Read the model definition and answer for the solid it produces. Units are mm, in the model's axes. A direction names the side the tool comes from. Give positions to 0.01 mm unless a question says otherwise; leave off trailing zeros. Order: outer loops, then holes, each group sorted by start corner. A loop starts at its lowest first (then second) coordinate and runs counter-clockwise, first axis right, second up.
Item 1: The mould has two halves that part along Z. Classify faces 1 (the face through (11.623, 3.738, -2.581)), 2 (the face through (8, 5.556, -4)), 3 (the face through (-3.86, 4.83, -5.04)): +Z half, -Z half, draft (parallel to the pull), parting line (faces both ways), or undercut.
Item 2: Given pin 1 Ø1 at (x, y) = (0, 8) entering from +Z; pin 2 Ø1 at (x, y) = (-7, 7) entering from +Z, each flat-ended and moving along its own axis, determine where each tip first touches the part or whether it passes through.
Item 3: A cutting plane is placed at D-D (y = 7.5). Write down the section's boundary in (x, z), plus the area to 3 significant figures.
Item 4: A cutting plane is placed at A-A (x = 0). Write down the section's boundary in (y, z) (3 decimals), plus the area to 3 significant figures.
Item 5: A cutting plane is placed at B-B (z = 0). Write down the section's boundary in (x, y) (3 decimals).
Item 6: A cutting plane is placed at C-C (y = 5). Write down the section's boundary in (x, z), plus the area to 3 significant figures.
Item 7: Which of the six approach directions +Z, -Z, +X, -X, +Y, -Y give full straight-line access (tool end or side, diameter ignored) to faces 4 (the face through (8.524, 4.751, 1.893)), 5 (the face through (-6, 0, 3))?
Item 8: Find the intervals of material crossed by line 1 along X through (y, z) = (4, 0); line 2 along X through (y, z) = (3.5, 0); line 3 along Y through (x, z) = (-4, 9.5), in increasing order.
from build123d import *

# Parameters (mm, degrees)
SKETCH1_R           = 8.73125
BOSS_EXTRUDE1_DEPTH = 9.525
SKETCH3_R           = 11.90625
BOSS_EXTRUDE2_DEPTH = 3.96875
BOSS_EXTRUDE3_START = -3.96875
SKETCH4_R           = 11.90625
BOSS_EXTRUDE3_DEPTH = 3.96875
SKETCH2_R           = 6.35
CUT_EXTRUDE2_DEPTH  = 20.345366451
FILLET2_R           = 3.5


with BuildPart() as part:
    # Sketch1 → Boss-Extrude1 (new body)
    with BuildSketch(Plane(origin=(0, 0, 0), x_dir=(1, 0, 0), z_dir=(0, 1, 0))):
        with Locations(Location((0, 0, 0), (0, 0, 90))):
            Circle(SKETCH1_R)
    extrude(amount=BOSS_EXTRUDE1_DEPTH)

    # Sketch3 → Boss-Extrude2 (add)
    with BuildSketch(Plane(origin=(0, 9.525, 0), x_dir=(1, 0, 0), z_dir=(0, 1, 0))):
        with Locations(Location((0, 0, 0), (0, 0, 270))):
            Circle(SKETCH3_R)
    extrude(amount=-BOSS_EXTRUDE2_DEPTH)

    # Sketch4 → Boss-Extrude3 (add)
    with BuildSketch(Plane(origin=(0, 0, 0), x_dir=(-1, 0, 0), z_dir=(0, -1, 0)).offset(BOSS_EXTRUDE3_START)):
        with Locations(Location((0, 0, 0), (0, 0, 270))):
            Circle(SKETCH4_R)
    extrude(amount=BOSS_EXTRUDE3_DEPTH)

    # Sketch2 → Cut-Extrude2 (cut, through all)
    with BuildSketch(Plane(origin=(0, 9.525, 0), x_dir=(1, 0, 0), z_dir=(0, 1, 0))):
        with Locations(Location((0, 0, 0), (0, 0, 270))):
            Circle(SKETCH2_R)
    extrude(amount=-CUT_EXTRUDE2_DEPTH, mode=Mode.SUBTRACT)

    # Fillet2
    fillet2_edges = [part.edges().sort_by_distance(p)[0] for p in [
        (0, 0, -11.90625),
        (0, 9.525, -11.90625),
    ]]
    fillet(fillet2_edges, radius=FILLET2_R)


solid = part.part
Response values:
1. face 1: parting line
1. face 2: draft
1. face 3: undercut
2. pin 1: stops at z = 11.58
2. pin 2: stops at z = 9.84
3. outline: circle Ø23.16 at (0, 0); hole circle Ø12.7 at (0, 0)
3. area: 295 mm2
4. outline: (0, -8.406) arc R3.5 ccw to (3.5, -11.906) - (3.969, -11.906) - (3.969, -8.731) - (5.556, -8.731) - (5.556, -11.906) - (6.025, -11.906) arc R3.5 ccw to (9.525, -8.406) - (9.525, -6.35) - (0, -6.35) - close; (0, 6.35) - (9.525, 6.35) - (9.525, 8.406) arc R3.5 ccw to (6.025, 11.906) - (5.556, 11.906) - (5.556, 8.731) - (3.969, 8.731) - (3.969, 11.906) - (3.5, 11.906) arc R3.5 ccw to (0, 8.406) - close
4. area: 85.3 mm2
5. outline: (-11.906, 3.5) arc R3.5 ccw to (-8.406, 0) - (-6.35, 0) - (-6.35, 9.525) - (-8.406, 9.525) arc R3.5 ccw to (-11.906, 6.025) - (-11.906, 5.556) - (-8.731, 5.556) - (-8.731, 3.969) - (-11.906, 3.969) - close; (6.35, 0) - (8.406, 0) arc R3.5 ccw to (11.906, 3.5) - (11.906, 3.969) - (8.731, 3.969) - (8.731, 5.556) - (11.906, 5.556) - (11.906, 6.025) arc R3.5 ccw to (8.406, 9.525) - (6.35, 9.525) - close
6. outline: circle Ø17.46 at (0, 0); hole circle Ø12.7 at (0, 0)
6. area: 113 mm2
7. face 4: none
7. face 5: +Z, -Z, +X, -X, -Y
8. line 1: x = -8.73 to -6.35, 6.35 to 8.73
8. line 2: x = -11.91 to -6.35, 6.35 to 11.91
8. line 3: y = 0.56 to 3.97, 5.56 to 8.96
